The listing builds one solid part. Answer for the finished solid, in the listing's coordinates (mm). Give positions to 0.01 mm unless a question says otherwise; leave off trailing zeros. Write each loop counter-clockwise with the first axis right and the second up, starting at its lowest first coordinate (ties: lowest second). Pieces come first, ordered by that corner, then holes. Notation, with made-up numbers: (-27, 38) - (9, 38) arc R23 cw to (9, 62) - close; hole circle Ø1 at (54.5, -26.75). An arc over 180 degrees is marked (long way). One line per question, with ' | ' between items. Start each with the question number.
1. The mould has two halves that part along X. Classify faces 1 (the face through (-0.439, 13.023, 1.521)), 2 (the face through (-15, 0, 1)), 3 (the face through (-4, 0, 0)): +X half, -X half, draft (parallel to the pull), parting line (faces both ways), or undercut.
2. A cutting plane is placed at A-A (x = 0). Determine the outline of the cut face in (y, z) (3 decimals).
3. Find the intervals of material crossed by L1, parallel to Y at x = 0, z = 1.3 (3 decimals); L2, parallel to Y at x = 1.75, z = 0.25; L3, parallel to X at y = 16.5, z = 0.4, in increasing order. Write a range as from..to.
4. A cutting plane is placed at B-B (y = 15). Determine the outline of the cut face in (x, z) (3 decimals), then the cut area to 4 significant figures.
5. A cutting plane is placed at C-C (z = 1.7). Determine the outline of the cut face in (x, y) (3 decimals), then the cut area to 3 significant figures.
6. A cutting plane is placed at D-D (y = 0.5). Determine the outline of the cut face in (x, z), then the cut area to 3 significant figures.
7. Given P1, Ø3, axis at x = 0, y = -1, coming from the +Z side, flat-ended and moving along its own axis, determine where the tip first touches the part or whether it passes through.
```python
from build123d import *

# Parameters (mm, degrees)
SKETCH_1_W          = 30
SKETCH_1_H          = 50
EXTRUDE_1_DEPTH     = 3
SKETCH_2_R          = 2.025
CUT_EXTRUDE_1_DEPTH = 4
SKETCH_3_R          = 2.025
CUT_EXTRUDE_2_DEPTH = 34
FILLET_1_R          = 2


with BuildPart() as part:
    # 草图1 → 凸台-拉伸1 (new body)
    with BuildSketch(Plane.XY):
        Rectangle(SKETCH_1_W, SKETCH_1_H)
    extrude(amount=EXTRUDE_1_DEPTH)

    # 草图2 → 切除-拉伸1 (cut)
    with BuildSketch(Plane.XY.offset(3)):
        with Locations((0, 15)):
            Circle(SKETCH_2_R)
    extrude(amount=-CUT_EXTRUDE_1_DEPTH, mode=Mode.SUBTRACT)

    # 草图3 → 切除-拉伸2 (cut)
    with BuildSketch(Plane.XY.offset(3)):
        with Locations((0, -1)):
            Circle(SKETCH_3_R)
        with Locations((0, -19)):
            Circle(SKETCH_3_R)
    extrude(amount=-CUT_EXTRUDE_2_DEPTH, mode=Mode.SUBTRACT)

    # 圆角1
    fillet_1_edges = [part.edges().sort_by_distance(p)[0] for p in [
        (15, -25, 1.5),
        (-15, -25, 1.5),
        (-15, 25, 1.5),
        (15, 25, 1.5),
    ]]
    fillet(fillet_1_edges, radius=FILLET_1_R)


solid = part.part
```
Determined:
1) face 1: undercut | face 2: -X half | face 3: draft
2) outline: (-25, 0) - (-21.025, 0) - (-21.025, 3) - (-25, 3) - close; (-16.975, 0) - (-3.025, 0) - (-3.025, 3) - (-16.975, 3) - close; (1.025, 0) - (12.975, 0) - (12.975, 3) - (1.025, 3) - close; (17.025, 0) - (25, 0) - (25, 3) - (17.025, 3) - close
3) L1: -25..-21.025, -16.975..-3.025, 1.025..12.975, 17.025..25 | L2: -25..-20.02, -17.98..-2.02, 0.02..13.98, 16.02..25 | L3: -15..-1.36, 1.36..15
4) outline: (-15, 0) - (-2.025, 0) - (-2.025, 3) - (-15, 3) - close; (2.025, 0) - (15, 0) - (15, 3) - (2.025, 3) - close | area: 77.85 mm2
5) outline: (-15, -23) arc R2 ccw to (-13, -25) - (13, -25) arc R2 ccw to (15, -23) - (15, 23) arc R2 ccw to (13, 25) - (-13, 25) arc R2 ccw to (-15, 23) - close; hole circle Ø4.05 at (0, -19); hole circle Ø4.05 at (0, -1); hole circle Ø4.05 at (0, 15) | area: 1,460 mm2
6) outline: (-15, 0) - (-1.36, 0) - (-1.36, 3) - (-15, 3) - close; (1.36, 0) - (15, 0) - (15, 3) - (1.36, 3) - close | area: 81.8 mm2
7) P1: through
